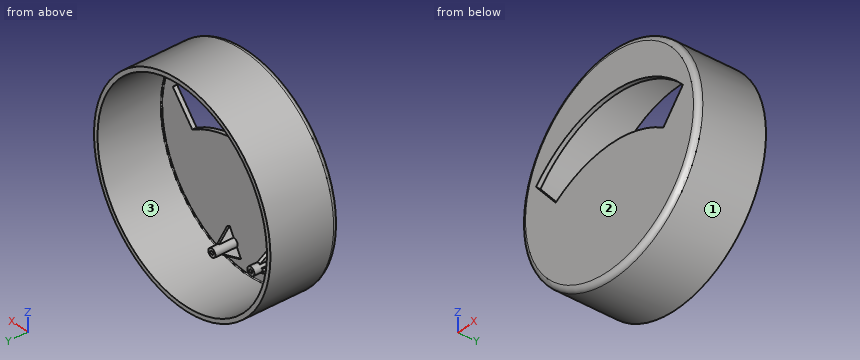
from build123d import *

# Parameters (mm, degrees)
F0_R             = 62.5
F1_DEPTH         = 40
F2_R             = 3
F3_T             = -2.5
F5_DEPTH         = 2.5
F6_R             = 2.5
F7_DEPTH         = 13
F8_R             = 1
F9_DEPTH         = 8
F12_DEPTH        = 1
F12_COPIES_COUNT = 3
F12_COPIES_ANGLE = 180
F15_DEPTH        = 1
F15_DEPTH_BACK   = 1
F15_COPIES_COUNT = 3
F15_COPIES_ANGLE = 180


# Not quite as in the source:
# - a pattern or mirror of a feature is missing from the dataset's text; its kind, count and spacing are read off the source's solid


with BuildPart() as f1:
    # F0 (on Front) → F1 (new body)
    with BuildSketch(Plane.XZ):
        Circle(F0_R)
    extrude(amount=F1_DEPTH)

    # F2
    f2_edges = [f1.edges().sort_by_distance(p)[0] for p in [
        (-62.5, -40, 0),
    ]]
    fillet(f2_edges, radius=F2_R)

    # F3
    f3_openings = [f1.faces().sort_by_distance(p)[0] for p in [
        (0, 0, 0),
    ]]
    offset(amount=F3_T, openings=f3_openings)

    # F4 (on face) → F5 (cut, through all)
    with BuildSketch(Plane.XZ.offset(40)):
        with BuildLine():
            ThreePointArc((52, 14.8614980554), (0, 38), (-52, 14.8614980554))
            Line((-52, 14.8614980554), (-38.1715582316, -1.3234958252))
            ThreePointArc((-38.1715582316, -1.3234958252), (0, 10), (38.1715582316, -1.3234958252))
            Line((38.1715582316, -1.3234958252), (52, 14.8614980554))
        make_face()
    extrude(amount=-F5_DEPTH, mode=Mode.SUBTRACT)

    # F6 (on face) → F7 (join)
    with BuildSketch(Plane(origin=(0, -37.5, 0), x_dir=(-1, 0, 0), z_dir=(0, 1, 0))):
        with Locations((-8.6170678389, -47.5194215546)):
            Circle(F6_R)
        with Locations((18.9575492455, -42.6572725799)):
            Circle(F6_R)
    extrude(amount=F7_DEPTH)

    # F8 (on face) → F9 (cut)
    with BuildSketch(Plane(origin=(0, -24.5, 0), x_dir=(-1, 0, 0), z_dir=(0, 1, 0))):
        with Locations((-8.6170678389, -47.5194215546)):
            Circle(F8_R)
        with Locations((18.9575492455, -42.6572725799)):
            Circle(F8_R)
    extrude(amount=-F9_DEPTH, mode=Mode.SUBTRACT)

    # F11 (on face) → F12 (join, symmetric)
    with BuildSketch(Plane(origin=(27.0393139988, 0, -15.6111552159), x_dir=(0, -1, 0), z_dir=(-0.8660254038, 0, 0.5))):
        Polygon((28.5, -34.84449232), (37.5, -34.84449232), (37.5, -28.84449232), align=None)
    f12 = extrude(amount=F12_DEPTH, both=True)

    # F12_copies: F12 ×3 about axis
    f12_copies_axis = Axis((8.617068, 0, -47.519422), (0, 1, 0))
    for i in range(1, F12_COPIES_COUNT):
        add(f12.rotate(f12_copies_axis, i * F12_COPIES_ANGLE / (F12_COPIES_COUNT - 1)))

    # F14 (on face) → F15 (join, two sides)
    with BuildSketch(Plane(origin=(-18.9575492455, 0, 0), x_dir=(0, -1, 0), z_dir=(-1, 0, 0))) as f15_sk:
        Polygon((28.5, -40.6572725799), (37.5, -40.6572725799), (37.5, -40.1572725799), (37.5, -34.6572725799), align=None)
    f15 = extrude(amount=F15_DEPTH) + extrude(f15_sk.sketch, amount=-F15_DEPTH_BACK)

    # F15_copies: F15 ×3 about axis
    f15_copies_axis = Axis((-18.957549, 0, -42.657273), (0, -1, 0))
    for i in range(1, F15_COPIES_COUNT):
        add(f15.rotate(f15_copies_axis, i * F15_COPIES_ANGLE / (F15_COPIES_COUNT - 1)))


solid = f1.part
Verification items for the finished model (mm, model axes). Face numbers are marked on the shaded views. Coordinates: 2 decimals unless noted, no trailing zeros. Order: outer loops, then holes, each group sorted by start corner. A loop starts at its lowest first (then second) coordinate and runs counter-clockwise, first axis right, second up. Notation, with made-up numbers: (47, 22.5) -> (56, 22.5) arc R34 ccw to (56, 61.5) -> close; hole circle Ø5 at (-4.75, 35.25). An arc over 180 degrees is marked (long way). Put each result on its own line as item: value. Start each with the question number.
1. Cross-section at C-C, the plane y = -12.5. Record the boundary of the cut face in (x, z).
2. Cross-section at A-A, the plane x = 0. Record the boundary of the cut face in (y, z), then the cut area to 3 significant figures.
3. Go/stop test with flat-tipped pins: pin 1 Ø1.7 at (y, z) = (-32, -48.5) entering from +X; pin 2 Ø4 at (x, z) = (8, -47.5) entering from +Y; pin 3 Ø3 at (x, z) = (36.5, -28) entering from +Y; pin 4 Ø6 at (x, z) = (7, 10) entering from -Y. Record where each tip stops, or that it passes through.
4. Cross-section at B-B, the plane y = -31. Record the boundary of the cut face in (x, z).
5. Material ranges on L1, parallel to Z at x = 1, y = -5.5; L2, parallel to X at y = -26, z = -2; L3, parallel to Y at x = -4.5, z = 9, recorded low to high. Write a range as [from, to].
6. Mould release check, pull along Z, two halves, no side actions. Record for the marked faces 1, 2 and 3: released by +Z, released by -Z, zero draft, split by the parting line, or undercut.
Computed:
1. outline: circle Ø125 at (0, 0); hole circle Ø120 at (0, 0)
2. outline: (-40, -59.5) arc R3 ccw to (-37, -62.5) -> (0, -62.5) -> (0, -60) -> (-37, -60) arc R0.5 cw to (-37.5, -59.5) -> (-37.5, 10) -> (-40, 10) -> close; (-40, 38) -> (-37.5, 38) -> (-37.5, 59.5) arc R0.5 cw to (-37, 60) -> (0, 60) -> (0, 62.5) -> (-37, 62.5) arc R3 ccw to (-40, 59.5) -> close
2. area: 426 mm2
3. pin 1: x = 40.44
3. pin 2: y = -24.5
3. pin 3: y = -37.5
3. pin 4: y = -40
4. outline: circle Ø125 at (0, 0); (-22.62, -43.66) -> (-21.25, -43.66) arc R2.5 ccw to (-19.96, -44.95) -> (-19.96, -46.32) -> (-17.96, -46.32) -> (-17.96, -44.95) arc R2.5 ccw to (-17.96, -40.37) -> (-17.96, -38.99) -> (-19.96, -38.99) -> (-19.96, -40.37) arc R2.5 ccw to (-21.25, -41.66) -> (-22.62, -41.66) -> close; (5.92, -50.19) -> (7.65, -51.19) -> (8.34, -50) arc R2.5 ccw to (10.1, -49.53) -> (11.29, -50.22) -> (12.29, -48.49) -> (11.1, -47.8) arc R2.5 ccw to (10.63, -46.04) -> (11.32, -44.84) -> (9.58, -43.84) -> (8.9, -45.04) arc R2.5 ccw to (6.61, -49) -> close; hole circle Ø120 at (0, 0); hole circle Ø2 at (-18.96, -42.66); hole circle Ø2 at (8.62, -47.52)
5. L1: [-62.49, -59.99], [59.99, 62.49]
5. L2: [-62.47, -59.97], [59.97, 62.47]
5. L3: [-40, -37.5]
6. face 1: split by the parting line
6. face 2: zero draft
6. face 3: undercut
